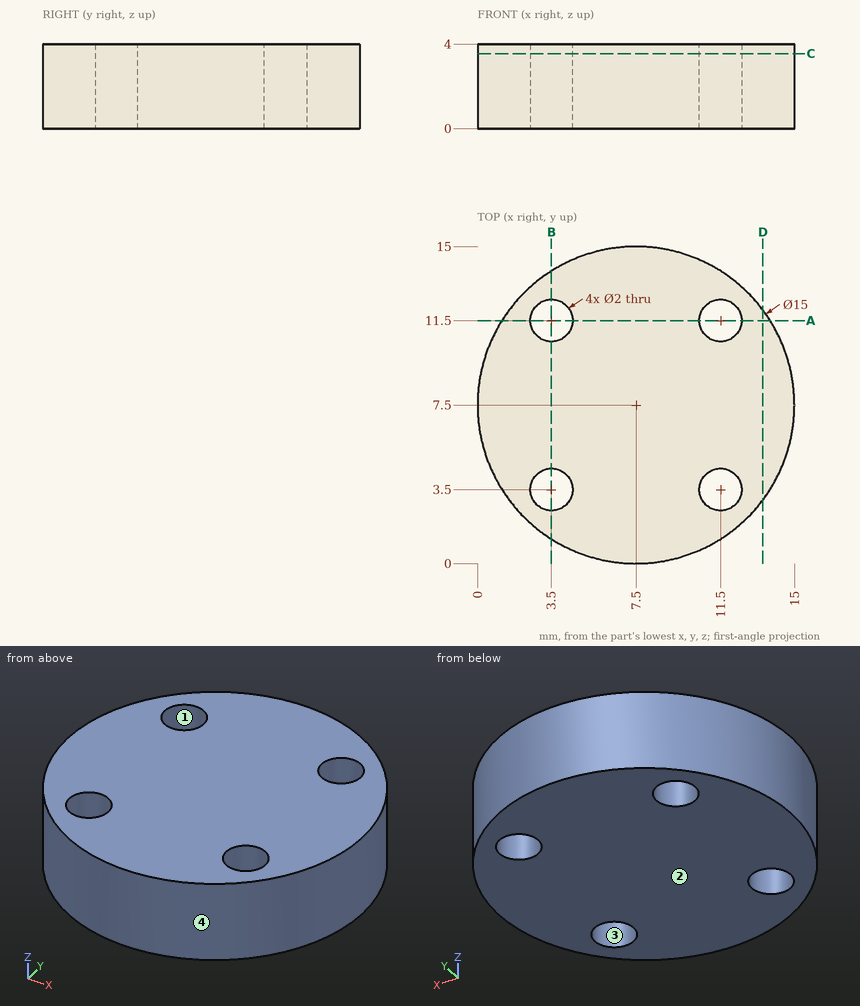
Part print with two shaded views. Sizes in mm from the minimum x, y, z corner. Round coordinates to 2 decimals unless told otherwise and drop trailing zeros. Loops run counter-clockwise (first coordinate to the right, second up) from the corner with the lowest first, then second, coordinate; pieces in that order, holes last. Notation, with made-up numbers: M 47.5,-26.75 L 106.5,-26.75 A11 ccw 106.5,-19.75 Z; hole C 42.25,25.25 d8. An arc over 180 degrees is marked long. Put each result on its own line as item: value. Start each with the question number.
Item 1: Cut at C-C (z = 3.55). List the corners of the cut face in (x, y), then the cut area to 3 significant figures.
Item 2: Drop flat-ended pins along their axis: P1, Ø2, axis at x = 4.5, z = 1, coming from the -Y side; P2, Ø2, axis at y = 10.5, z = 2.5, coming from the -X side; P3, Ø1, axis at x = 11.5, z = 1.5, coming from the +Y side. Give the stop position or say it passes through.
Item 3: Mould opens along Y. For the marked faces 1, 2, 3 and 4 say: released by +Y, released by -Y, zero draft, split by the parting line, or undercut.
Item 4: Drill centre lines: line 1 along X through (y, z) = (3.5, 2.1); line 2 along Y through (x, z) = (3, 3.7); line 3 along X through (y, z) = (11.25, 2.7). Where is each one in solid material? Low to high.
Item 5: Cut at D-D (x = 13.5). List the corners of the cut face in (y, z), then the cut area to 3 significant figures.
Item 6: Cut at A-A (y = 11.5). List the corners of the cut face in (x, z), then the cut area to 3 significant figures.
Answer block:
1. outline: C 7.5,7.5 d15; hole C 3.5,3.5 d2; hole C 3.5,11.5 d2; hole C 11.5,3.5 d2; hole C 11.5,11.5 d2
1. area: 164 mm2
2. P1: y = 0.27
2. P2: x = 0.27
2. P3: y = 14.13
3. face 1: undercut
3. face 2: zero draft
3. face 3: undercut
3. face 4: split by the parting line
4. line 1: 1.16 to 2.5, 4.5 to 10.5, 12.5 to 13.84
4. line 2: 1.5 to 2.63, 4.37 to 10.63, 12.37 to 13.5
4. line 3: 1 to 2.53, 4.47 to 10.53, 12.47 to 14
5. outline: M 3,0 L 12,0 L 12,4 L 3,4 Z
5. area: 36.0 mm2
6. outline: M 1.16,0 L 2.5,0 L 2.5,4 L 1.16,4 Z; M 4.5,0 L 10.5,0 L 10.5,4 L 4.5,4 Z; M 12.5,0 L 13.84,0 L 13.84,4 L 12.5,4 Z
6. area: 34.8 mm2
